Autodesk Inventor part; units mm, degrees
ref_plane "YZ Plane" through (0, 0, 0) normal (1, 0, 0) x (0, 1, 0)
ref_plane "XZ Plane" through (0, 0, 0) normal (0, 1, 0) x (-1, 0, 0)
ref_plane "XY Plane" through (0, 0, 0) normal (0, 0, 1) x (1, 0, 0)
sketch "Skizze1" plane through (0, 0, 0) normal (0, 1, 0) x (-1, 0, 0)
  circle A0 centre (0, 0) radius 7.5
  dimension "d0" = 15
extrude "Extrusion1" add sketch "Skizze1" along normal blind 40
sketch "Skizze2" plane through (0, 40, 0) normal (0, 1, 0) x (1, 0, 0)
  arc A0 (2, 1.6613) -> (2, -1.6613) centre (0, 0) ccw
  line L0 (2, -1.6613) -> (2, 1.6613)
  dimension "d3" = 5.2
  dimension "d4" = 4.6
extrude "Extrusion2" cut sketch "Skizze2" against normal blind 15
sketch "Skizze3" plane through (0, 0, 0) normal (1, 0, 0) x (0, 1, 0)
  line L0 (-8, 0) -> (48, 0) construction
  line L1 (40, -7.5) -> (40, 7.5)
  line L2 (0, 7.5) -> (0, -7.5)
  point P0 (0, 0)
  point P1 (18.5, 0)
  dimension "d7" = 21.5
hole "Bohrung1" at (0, 18.5, 0) direction (-1, 0, 0) diameter 4 end through all both
properties part number "Motor_Spiral"
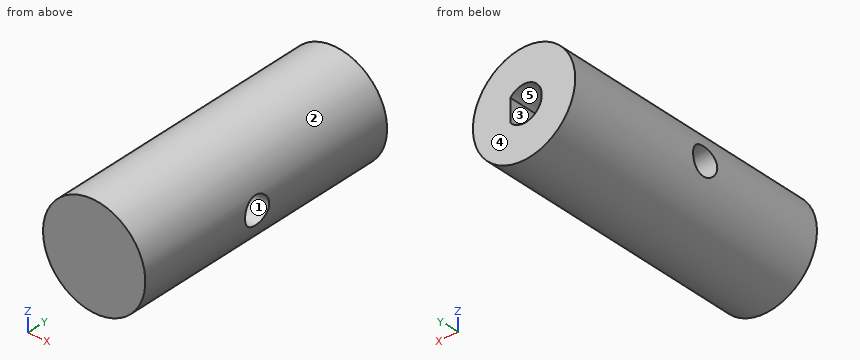
Geometry: final body of the model. Coordinates: model frame, mm. Face numbers are marked on the shaded views. A direction names the side the tool comes from. Coordinates: 2 decimals unless noted, no trailing zeros. Order: outer loops, then holes, each group sorted by start corner. A loop starts at its lowest first (then second) coordinate and runs counter-clockwise, first axis right, second up. Notation, with made-up numbers: (79.5, 52.25) -> (103.5, 52.25) arc R29 ccw to (103.5, 91.25) -> close; hole circle Ø3 at (-6.75, -5.5). An arc over 180 degrees is marked (long way). Use CSV: the item, a comma, the result in double quotes.
1) Line query: line 1 (Z direction, x = 0, y = 36.25); line 2 (Y direction, x = 2.25, z = 0); line 3 (Y direction, x = -4, z = -1.5). Output: solid intervals per line, ascending.
Findings:
line 1,"z = -7.5 to -2.6, 2.6 to 7.5"
line 2,"y = 0 to 16.5, 20.5 to 40"
line 3,"y = 0 to 17.18, 19.82 to 40"
2) Section B-B on x = 0. Output: boundary loops of the cut face in (y, z).
Findings:
outline,"(0, -7.5) -> (40, -7.5) -> (40, -2.6) -> (25, -2.6) -> (25, 2.6) -> (40, 2.6) -> (40, 7.5) -> (0, 7.5) -> close; hole circle Ø4 at (18.5, 0)"
3) Section A-A on z = 0. Output: boundary loops of the cut face in (x, y), then the cut area to 3 significant figures.
Findings:
outline,"(-7.5, 0) -> (7.5, 0) -> (7.5, 16.5) -> (-7.5, 16.5) -> close; (-7.5, 20.5) -> (7.5, 20.5) -> (7.5, 40) -> (2, 40) -> (2, 25) -> (-2.6, 25) -> (-2.6, 40) -> (-7.5, 40) -> close"
area,"471 mm^2"
4) Mould query, pull axis X, two halves, no side actions, for the marked faces 1, 2 and 3. Classes: +X half, -X half, draft (parallel to the pull), parting line (faces both ways), or undercut.
Findings:
face 1,"draft"
face 2,"parting line"
face 3,"undercut"
5) Pin query (flat end, axial travel): pin 1 Ø5 at (x, y) = (3, 20) entering from +Z; pin 2 Ø4 at (x, y) = (5, 20) entering from -Z. Return the tip coordinate at first contact, or that it passes through.
Findings:
pin 1,"stops at z = 7.48"
pin 2,"stops at z = -6.87"
6) Section D-D on x = 4.5. Output: boundary loops of the cut face in (y, z).
Findings:
outline,"(0, -6) -> (40, -6) -> (40, 6) -> (0, 6) -> close; hole circle Ø4 at (18.5, 0)"
7) Section C-C on y = 18.5. Output: boundary loops of the cut face in (x, z).
Findings:
outline,"(-7.23, -2) arc R7.5 ccw to (7.23, -2) -> close; (-7.23, 2) -> (7.23, 2) arc R7.5 ccw to start"
8) Access query for the marked faces 4 and 5. Directions: +Z, -Z, +X, -X, +Y, -Y. A direction counts if a zero-diameter tool reaches every point of the face in a straight line with its end or side. Return the directions, or none.
Findings:
face 4,"+Z, -Z, +X, -X, +Y"
face 5,"+Y"
